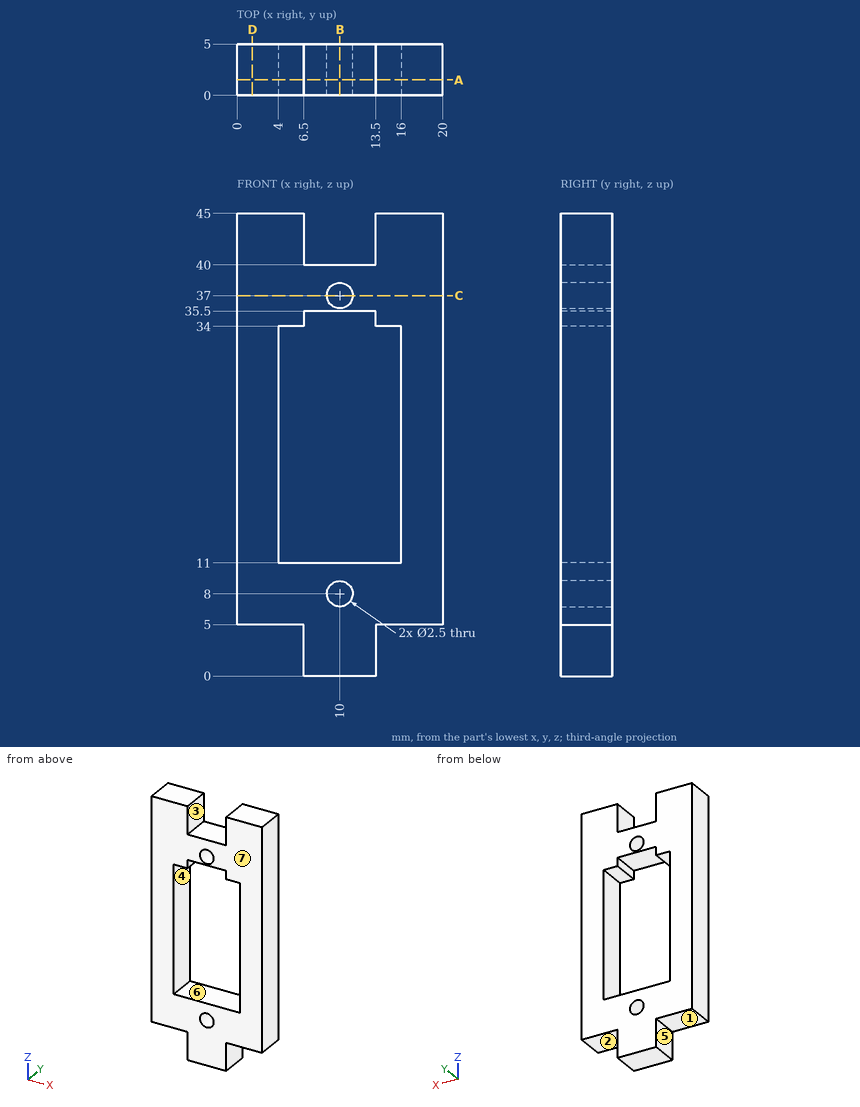
Design review of the part shown in the three views and the two pictorial views. Dimensions are in mm from the part's minimum x, y and z. A direction names the side the tool comes from. Give positions to 0.01 mm unless a question says otherwise; leave off trailing zeros. Loops run counter-clockwise (first coordinate to the right, second up) from the corner with the lowest first, then second, coordinate; pieces in that order, holes last. Notation, with made-up numbers: M -35,28.25 L -14,28.25 A31 cw -14,58.25 Z; hole C 68.25,59 d9. An arc over 180 degrees is marked long. Put each result on its own line as item: value. Start each with the question number.
(1) Add section C-C, the plane z = 37. Write out the cut boundary in (x, y).
(2) Add section B-B, the plane x = 10. Write out the cut boundary in (y, z), then the cut area to 3 significant figures.
(3) The part is to be moulded in two halves that separate along X. For the marked faces 5, 6 and 7, say which applies: +X half, -X half, draft (parallel to the pull), parting line (faces both ways), or undercut.
(4) Wall thickness on L1, parallel to X at y = 2.15, z = 34.5; L2, parallel to X at y = 2.15, z = 8; L3, parallel to Z at x = 5.5, y = 0.75: over which ranges is each line inside the solid? List them lowest first.
(5) For pin 1 (1.5 mm diameter, centred on x = 8, y = 3.5, fed in from +Z); pin 2 (0.8 mm diameter, centred on x = 14.5, y = 3.5, fed in from -Z); pin 3 (2 mm diameter, centred on x = 10, z = 8, fed in from -Y); pin 4 (3 mm diameter, centred on x = 10, z = 37, fed in from +Y), all flat-tipped, find the tip position at first contact; note any pin that passes through.
(6) Machinability: for the marked faces 1, 2, 3 and 4, which of the approach directions +Z, -Z, +X, -X, +Y, -Y give a long, thin tool a straight path to every point of the face, cutting with its end or side? Answer none if there is none.
(7) Add section A-A, the plane y = 1.5. Write out the cut boundary in (x, z).
(8) Add section D-D, the plane x = 1.5. Write out the cut boundary in (y, z), then the cut area to 3 significant figures.
Result:
1. outline: M 0,0 L 8.75,0 L 8.75,5 L 0,5 Z; M 11.25,0 L 20,0 L 20,5 L 11.25,5 Z
2. outline: M 0,0 L 5,0 L 5,6.75 L 0,6.75 Z; M 0,9.25 L 5,9.25 L 5,11 L 0,11 Z; M 0,35.5 L 5,35.5 L 5,35.75 L 0,35.75 Z; M 0,38.25 L 5,38.25 L 5,40 L 0,40 Z
2. area: 52.5 mm^2
3. face 5: -X half
3. face 6: undercut
3. face 7: draft
4. L1: x = 0 to 6.5, 13.5 to 20
4. L2: x = 0 to 8.75, 11.25 to 20
4. L3: z = 5 to 11, 34 to 45
5. pin 1: stops at z = 40
5. pin 2: stops at z = 5
5. pin 3: passes through
5. pin 4: stops at y = 5
6. face 1: -Z, -X, +Y, -Y
6. face 2: -Z, +X, +Y, -Y
6. face 3: +Z, +Y, -Y
6. face 4: +Y, -Y
7. outline: M 0,5 L 6.5,5 L 6.5,0 L 13.5,0 L 13.5,5 L 20,5 L 20,45 L 13.5,45 L 13.5,40 L 6.5,40 L 6.5,45 L 0,45 Z; hole M 4,11 L 16,11 L 16,34 L 13.5,34 L 13.5,35.5 L 6.5,35.5 L 6.5,34 L 4,34 Z; hole C 10,8 d2.5; hole C 10,37 d2.5
8. outline: M 0,5 L 5,5 L 5,45 L 0,45 Z
8. area: 200 mm^2
